Autodesk Inventor part; units mm, degrees
ref_plane "YZ Plane" through (0, 0, 0) normal (1, 0, 0) x (0, 1, 0)
ref_plane "XZ Plane" through (0, 0, 0) normal (0, 1, 0) x (-1, 0, 0)
ref_plane "XY Plane" through (0, 0, 0) normal (0, 0, 1) x (1, 0, 0)
sketch "Sketch1" plane through (0, 0, 0) normal (1, 0, 0) x (0, 1, 0)
  line L0 (0, 18) -> (5.825, 18) construction
  line L1 (0, 0) -> (7.3998, 0) construction
  line L2 (0, 12.5) -> (0, 0) construction
  line L3 (7.3998, 0) -> (9, 0) construction
  line L4 (9, 0) -> (9, 18)
  line L5 (9, 18) -> (9, 18)
  line L6 (9, 18) -> (9, 20)
  line L7 (9, 20) -> (7, 20)
  line L8 (7, 20) -> (7, 18)
  line L9 (5.825, 18) -> (7, 18) construction
  line L10 (5.825, 18) -> (7.3998, 0) construction
  line L11 (6, 18) -> (7, 18)
  line L12 (6, 16) -> (7.3998, 0)
  line L13 (9, 0) -> (7.3998, 0)
  line L14 (6, 18) -> (6, 16)
  point P0 (2.25, 0)
  dimension "d2" = 18
  dimension "d12" = 2
  dimension "d14" = 0
  dimension "d16" = 2
  dimension "d17" = 7
  dimension "d35" = 95
  dimension "d36" = 9
  dimension "d57" = 2
  dimension "d60" = 6
revolve "Revolution1" add sketch "Sketch1" angle 360 about axis through (0, 0, 12.5) along (0, 0, -1)
sketch "Sketch3" plane through (0, 0, 0) normal (1, 0, 0) x (0, 1, 0)
  line L0 (14, 0) -> (14, 18)
  line L1 (14, 18) -> (7.3998, 18)
  line L2 (14, 0) -> (7.3998, 0)
  line L3 (-7.3998, 0) -> (7.3998, 0)
  line L4 (7.3998, 0) -> (7.3998, 18)
  line L5 (-6, 18) -> (6, 18)
  point P0 (0, 0)
  dimension "d28" = 14
extrude "Extrusion1" add sketch "Sketch3" along normal mid plane 8
sketch "Sketch4" plane through (-4, 0, 0) normal (-1, 0, 0) x (0, 0, 1)
  circle A0 centre (5.5, 10.25) radius 1.6
  circle A1 centre (12.5, 10.25) radius 1.6
  line L0 (5.5, 10.25) -> (12.5, 10.25) construction
  line L1 (18, 14) -> (0, 14) construction
  point P0 (0, 0)
  point P1 (17, 10.25)
  point P2 (9, 10.25)
  point P3 (9, 14)
  dimension "d29" = 3.2
  dimension "d30" = 3.2
  dimension "d31" = 7
  dimension "d34" = 3.75
extrude "Extrusion2" cut sketch "Sketch4" against normal blind 10
sketch "Sketch5" plane through (4, 0, 0) normal (1, 0, 0) x (0, 0, -1)
  circle A0 centre (-5.5, 10.25) radius 1.6
  circle A1 centre (-12.5, 10.25) radius 1.6
  line L0 (0, 8.0623) -> (-18, 8.0623)
  line L1 (-20.496, 14) -> (-16.5, 14)
  line L2 (-16.5, 14) -> (-16.5, 8.0623)
  line L3 (-16.5, 8.0623) -> (-20.496, 8.0623)
  line L4 (-20.496, 8.0623) -> (-20.496, 14)
  line L5 (0, 14) -> (-1.5, 14)
  line L6 (-1.5, 14) -> (-1.5, 8.0623)
  line L7 (-1.5, 8.0623) -> (0, 8.0623)
  line L8 (0, 8.0623) -> (0, 14)
  line L9 (0, 14) -> (-18, 14)
  point P0 (0, 0)
  dimension "d47" = 15
  dimension "d49" = 4
  dimension "d50" = 4
extrude "Extrusion3" cut sketch "Sketch5" against normal blind 10 contours L0 L6 L5 L8 | L0 L3 L4 L1 L2
equation "\"d49\" = d50"
properties part number "brush holder v4"
Read the model definition and answer for the solid it produces. Units are mm, in the model's axes. A direction names the side the tool comes from. Round coordinates to 2 decimals unless told otherwise and drop trailing zeros. Write each loop counter-clockwise with the first axis right and the second up, starting at its lowest first coordinate (ties: lowest second). Pieces come first, ordered by that corner, then holes. Notation, with made-up numbers: M 2.25,-27.75 L 26.25,-27.75 A35 cw 26.25,7.25 Z; hole C 49.25,82.5 d1. An arc over 180 degrees is marked long. One line per item, written item: value.
Q1. Find section C-C on y = 0. Write down the section's boundary in (x, z).
Data:
outline: M -9,0 L -7.4,0 L -6,16 L -6,18 L -7,18 L -7,20 L -9,20 Z; M 6,16 L 7.4,0 L 9,0 L 9,20 L 7,20 L 7,18 L 6,18 Z
Q2. For a pull along Y with two mould halves and no side action, classify faces 5 (the cylindrical face through (-0.06, 8.69, 5.15)), 6 (the flat face through (0, 8.062, 1)), 7 (the flat face through (0, 11, 16.5)) as +Y half, -Y half, draft (parallel to the pull), parting line (faces both ways), or undercut.
Data:
face 5: undercut
face 6: +Y half
face 7: draft
Q3. Find section A-A on x = 0. Write down the section's boundary in (y, z).
Data:
outline: M -9,0 L -7.4,0 L -6,16 L -6,18 L -7,18 L -7,20 L -9,20 Z; M 6,16 L 7.4,0 L 8.06,0 L 8.06,1.5 L 14,1.5 L 14,16.5 L 8.06,16.5 L 8.06,20 L 7,20 L 7,18 L 6,18 Z; hole C 10.25,5.5 d3.2; hole C 10.25,12.5 d3.2
Q4. Which of the six approach directions +Z, -Z, +X, -X, +Y, -Y give full straight-line access (tool end or side, diameter ignored) to faces 1 (the flat face through (-4, 11, 9)), 2 (the flat face through (0, 11, 1.5)), 3 (the flat face through (4, 11, 9)), 4 (the flat face through (2, 6, 18))?
Data:
face 1: +Z, -Z, -X, +Y
face 2: -Z, +X, -X, +Y
face 3: +Z, -Z, +X, +Y
face 4: +Z
Q5. Find section D-D on y = 11.25. Write down the section's boundary in (x, z), plus the area to 3 significant figures.
Data:
outline: M -4,1.5 L 4,1.5 L 4,4.25 L -4,4.25 Z; M -4,6.75 L 4,6.75 L 4,11.25 L -4,11.25 Z; M -4,13.75 L 4,13.75 L 4,16.5 L -4,16.5 Z
area: 80.0 mm2
Q6. Flat-ended cylindrical pins translate along their axes: pin 1 Ø6.5 at (y, z) = (11.5, 5.5) entering from -X; pin 2 Ø4 at (x, z) = (1, 7) entering from -Y; pin 3 Ø3 at (y, z) = (11, 6.5) entering from +X; pin 4 Ø1 at (x, z) = (-1.5, 19) entering from +Y. Find the tip coordinate at first contact, or state that the pin passes through.
Data:
pin 1: x = -4
pin 2: y = -9
pin 3: x = 4
pin 4: y = 8.06
Q7. Straight lines are drawn through the part: line 1 (Y direction, x = 1, z = 5.5); line 2 (X direction, y = 0, z = 16.7); line 3 (X direction, y = 0, z = 18.75). For each, find the intervals that lie inside material, in ascending order. Write a range as [from, to].
Data:
line 1: [-8.94, -6.85], [6.85, 8.65], [11.85, 14]
line 2: [-9, -6], [6, 9]
line 3: [-9, -7], [7, 9]
Q8. Find section B-B on z = 12.5. Write down the section's boundary in (x, y).
Data:
outline: M -4,8.06 A9 ccw long 4,8.06 L 4,8.65 L -4,8.65 Z; M -4,11.85 L 4,11.85 L 4,14 L -4,14 Z; hole C 0,0 d12.61
